Model file for the job. Use its own axes, mm. Face numbers are marked on the shaded views. A direction names the side the tool comes from. Round coordinates to 2 decimals unless told otherwise and drop trailing zeros. Loops run counter-clockwise (first coordinate to the right, second up) from the corner with the lowest first, then second, coordinate; pieces in that order, holes last. Notation, with made-up numbers: M 85,14.5 L 101,14.5 A17 cw 101,36.5 Z; hole C 78.5,47 d9. An arc over 180 degrees is marked long. Answer in a Markdown table with one row per item.
from build123d import *

# Parameters (mm, degrees)
MAIN_DEPTH                   = 24
SK_RECESS_R                  = 21
RECESS_DEPTH                 = 4
NUT_DEPTH                    = 83
SK_HOLE1_R                   = 2.5
HOLE1_DEPTH                  = 5
SK_HOLE_T_R                  = 4
HOLE_T_DEPTH                 = 17
SK_HOLE2_R                   = 4
HOLE2_DEPTH                  = 13
SK_HOLE3_R                   = 4
HOLE3_DEPTH                  = 16
SKETCH1_R                    = 3.3
THRUHOLES_DEPTH              = 113.841703284
SK_PRONG_GRV_W               = 8.5
SK_PRONG_GRV_H               = 119
PRONG_GRV_DEPTH              = 9
SK_HOLE4_R                   = 2.5
HOLE4_DEPTH                  = 5
GRV_REACH                    = 119.133
F_32_40SWITCHCHAMFER_SIZE    = 4.5
SKETCH5_W                    = 0.7
SKETCH5_H                    = 5
F_32_40SWITCHCUTDETAIL_DEPTH = 105.905910224
EXTRUDE1_START               = 5
SKETCH6_R                    = 2.5
EXTRUDE1_DEPTH               = 5
SKETCH9_R                    = 2.5
HOLE_5_DEPTH                 = 5


with BuildPart() as part:
    # sk-main → main (new, symmetric)
    with BuildSketch(Plane.XY):
        Polygon((0, -36), (83, -36), (83, 36), (0, 36), (0, 59.5), (-15, 59.5), (-15, -59.5), (0, -59.5), align=None)
    extrude(amount=MAIN_DEPTH, both=True)

    # sk-recess → recess (cut)
    with BuildSketch(Plane(origin=(83, 0, 0), x_dir=(0, 0, -1), z_dir=(1, 0, 0))):
        with Locations(Location((0, 0, 0), (0, 0, 90))):
            Circle(SK_RECESS_R)
    extrude(amount=-RECESS_DEPTH, mode=Mode.SUBTRACT)

    # sk-NUT → NUT (cut)
    with BuildSketch(Plane(origin=(83, 0, 0), x_dir=(0, 0, -1), z_dir=(1, 0, 0))):
        with BuildLine():
            Line((-21.622875656, 16.2), (-24, 16.2))
            Line((-24, 16.2), (-24, 13.2))
            Line((-24, 13.2), (-21.622875656, 13.2))
            ThreePointArc((-21.622875656, 13.2), (-18.3, 14.7), (-21.622875656, 16.2))
        make_face()
        with BuildLine():
            Line((-21.622875656, -13.2), (-24, -13.2))
            Line((-24, -13.2), (-24, -16.2))
            Line((-24, -16.2), (-21.622875656, -16.2))
            ThreePointArc((-21.622875656, -16.2), (-18.3, -14.7), (-21.622875656, -13.2))
        make_face()
        with BuildLine():
            Line((21.622875656, 13.2), (24, 13.2))
            Line((24, 13.2), (24, 16.2))
            Line((24, 16.2), (21.622875656, 16.2))
            ThreePointArc((21.622875656, 16.2), (18.3, 14.7), (21.622875656, 13.2))
        make_face()
        with BuildLine():
            Line((21.622875656, -13.2), (24, -13.2))
            Line((24, -13.2), (24, -16.2))
            Line((24, -16.2), (21.622875656, -16.2))
            ThreePointArc((21.622875656, -16.2), (18.3, -14.7), (21.622875656, -13.2))
        make_face()
    extrude(amount=-NUT_DEPTH, mode=Mode.SUBTRACT)

    # sk-hole1 → hole1 (cut)
    with BuildSketch(Plane(origin=(83, 0, 0), x_dir=(0, 0, -1), z_dir=(1, 0, 0))):
        with Locations(Location((-14, 29, 0), (0, 0, 90))):
            Circle(SK_HOLE1_R)
    extrude(amount=-HOLE1_DEPTH, mode=Mode.SUBTRACT)

    # sk-hole_t → hole_t (cut)
    with BuildSketch(Plane(origin=(83, 0, 0), x_dir=(0, 0, -1), z_dir=(1, 0, 0))):
        with Locations(Location((-16, -28, 0), (0, 0, 90))):
            Circle(SK_HOLE_T_R)
        with Locations(Location((16, 28, 0), (0, 0, 90))):
            Circle(SK_HOLE_T_R)
    extrude(amount=-HOLE_T_DEPTH, mode=Mode.SUBTRACT)

    # sk-hole2 → hole2 (cut)
    with BuildSketch(Plane(origin=(0, 36, 0), x_dir=(-1, 0, 0), z_dir=(0, 1, 0))):
        with Locations((-25, -16)):
            Circle(SK_HOLE2_R)
        with Locations((-25, 16)):
            Circle(SK_HOLE2_R)
    extrude(amount=-HOLE2_DEPTH, mode=Mode.SUBTRACT)

    # sk-hole3 → hole3 (cut)
    with BuildSketch(Plane(origin=(0, 0, -24), x_dir=(-1, 0, 0), z_dir=(0, 0, -1))):
        with Locations((-34, 28)):
            Circle(SK_HOLE3_R)
        with Locations((-34, -28)):
            Circle(SK_HOLE3_R)
    hole3 = extrude(amount=-HOLE3_DEPTH, mode=Mode.SUBTRACT)

    # Mirror1: hole3 across plane
    add(hole3.mirror(Plane.XY), mode=Mode.SUBTRACT)

    # Sketch1 → ThruHoles (cut, through all)
    with BuildSketch(Plane.XY.offset(24)):
        with Locations((34, 28)):
            Circle(SKETCH1_R)
        with Locations((34, -28)):
            Circle(SKETCH1_R)
    extrude(amount=-THRUHOLES_DEPTH, mode=Mode.SUBTRACT)

    # sk-prong_grv → prong_grv (cut, symmetric)
    with BuildSketch(Plane.XY):
        with Locations((-10.75, 0)):
            Rectangle(SK_PRONG_GRV_W, SK_PRONG_GRV_H)
    extrude(amount=PRONG_GRV_DEPTH, both=True, mode=Mode.SUBTRACT)

    # sk-hole4 → hole4 (cut)
    with BuildSketch(Plane.XZ.offset(36)):
        with Locations((45, 14)):
            Circle(SK_HOLE4_R)
        with Locations((71, -14)):
            Circle(SK_HOLE4_R)
    extrude(amount=-HOLE4_DEPTH, mode=Mode.SUBTRACT)

    # grv: up to this face of the body (flat: up to its plane)
    grv_end = Plane(part.part.faces().sort_by_distance((0, 47.75, 0))[0])
    # sk-grv → grv (cut, up to the picked face)
    with BuildSketch(Plane(origin=(83, 0, 0), x_dir=(0, 0, -1), z_dir=(1, 0, 0)), mode=Mode.PRIVATE) as grv_sk1:
        Polygon((-2.5, 36), (-2.5, 27.3), (-3.1, 27.020215405), (-3.1, 23), (3.1, 23), (3.1, 27.020215405), (2.5, 27.3), (2.5, 36), align=None)
    grv_tool1 = split(extrude(grv_sk1.sketch, amount=-GRV_REACH, mode=Mode.PRIVATE), bisect_by=grv_end, keep=Keep.BOTH, mode=Mode.PRIVATE)
    # sk-grv → grv (cut, up to the picked face)
    with BuildSketch(Plane(origin=(83, 0, 0), x_dir=(0, 0, -1), z_dir=(1, 0, 0)), mode=Mode.PRIVATE) as grv_sk2:
        Polygon((3.1, -23), (3.1, -27.020215405), (2.5, -27.3), (2.5, -36), (-2.5, -36), (-2.5, -27.3), (-3.1, -27.020215405), (-3.1, -23), align=None)
    grv_tool2 = split(extrude(grv_sk2.sketch, amount=-GRV_REACH, mode=Mode.PRIVATE), bisect_by=grv_end, keep=Keep.BOTH, mode=Mode.PRIVATE)
    add(grv_tool1.solids().sort_by(Axis((83, 29.184807, 0), (-1, 0, 0)))[0], mode=Mode.SUBTRACT)
    add(grv_tool2.solids().sort_by(Axis((83, -29.184807, 0), (-1, 0, 0)))[0], mode=Mode.SUBTRACT)

    # 32-40SwitchChamfer
    f_32_40switchchamfer_edges = [part.edges().sort_by_distance(p)[0] for p in [
        (41.5, 36, -2.5),
        (41.5, 36, 2.5),
        (41.5, -36, 2.5),
        (41.5, -36, -2.5),
    ]]
    chamfer(f_32_40switchchamfer_edges, length=F_32_40SWITCHCHAMFER_SIZE)

    # Sketch5 → 32-40SwitchCutDetail (cut, through all)
    with BuildSketch(Plane(origin=(0, 0, 0), x_dir=(0, 0, -1), z_dir=(1, 0, 0))):
        with Locations((-23.65, 14.7)):
            Rectangle(SKETCH5_W, SKETCH5_H)
        with Locations((23.65, 14.7)):
            Rectangle(SKETCH5_W, SKETCH5_H)
        with Locations((23.65, -14.7)):
            Rectangle(SKETCH5_W, SKETCH5_H)
        with Locations((-23.65, -14.7)):
            Rectangle(SKETCH5_W, SKETCH5_H)
    extrude(amount=F_32_40SWITCHCUTDETAIL_DEPTH, mode=Mode.SUBTRACT)

    # Sketch6 → Extrude1 (add)
    with BuildSketch(Plane.XZ.offset(31).offset(EXTRUDE1_START)):
        with Locations((71, -14)):
            Circle(SKETCH6_R)
    extrude(amount=-EXTRUDE1_DEPTH)

    # Sketch9 → Hole 5 (cut)
    with BuildSketch(Plane.XZ.offset(36)):
        with Locations((71, -14)):
            Circle(SKETCH9_R)
    extrude(amount=-HOLE_5_DEPTH, mode=Mode.SUBTRACT)


solid = part.part
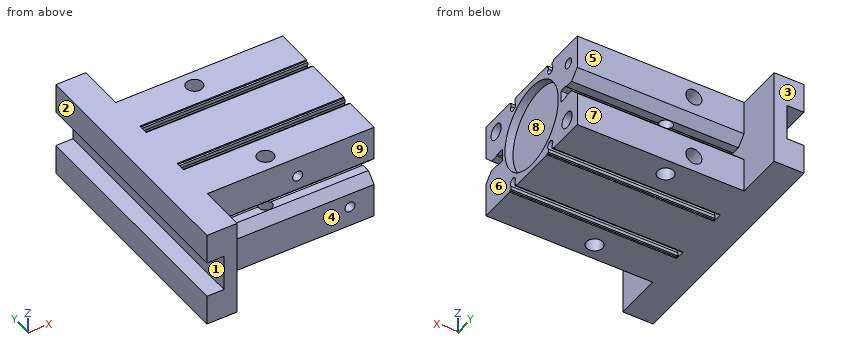
1. Saw through at A-A (z = 0). Write the cut outline in (x, y), and give its area (3 significant figures).
Verdict:
| item | result |
|---|---|
| outline | M -6.5,-59.5 L 0,-59.5 L 0,-23 L 83,-23 L 83,-21 L 79,-21 L 79,21 L 83,21 L 83,23 L 0,23 L 0,59.5 L -6.5,59.5 Z |
| area | 4,420 mm² |
2. Mould opens along Y. For the marked faces 6, 7, 8 and 9 say: +Y half, -Y half, draft (parallel to the pull), parting line (faces both ways), or undercut.
Verdict:
| item | result |
|---|---|
| face 6 | draft |
| face 7 | +Y half |
| face 8 | undercut |
| face 9 | -Y half |
3. Saw through at C-C (y = -50.5). Write the cut outline in (x, z), and give its area (3 significant figures).
Verdict:
| item | result |
|---|---|
| outline | M -15,-24 L 0,-24 L 0,24 L -15,24 L -15,9 L -6.5,9 L -6.5,-9 L -15,-9 Z |
| area | 567 mm² |
4. Saw through at B-B (x = 71). State how many separate pieces and enclosed holes the cut face has, and give its area (3 significant figures).
Verdict:
| item | result |
|---|---|
| separate pieces | 1 |
| enclosed holes | 2 |
| area | 3,070 mm² |
5. Tool access for the marked faces 1, 2, 3, 4 and 5: list every direction of +Z, -Z, +X, -X, +Y, -Y with a clear straight run to the whole face (end or side of a thin tool).
Verdict:
| item | result |
|---|---|
| face 1 | -X, +Y, -Y |
| face 2 | +Z, -Z, -X, +Y, -Y |
| face 3 | +Z, -Z, +X, -X, +Y |
| face 4 | +Z, -Z, +X, -Y |
| face 5 | +Z, -Z, +X, +Y |
6. Wall check: probe 1 along Z at (x, y) = (25, 30.5); probe 2 along Y at (x, z) = (34, -14.25); probe 3 along Z at (x, y) = (81.25, 0). Give the ranges that are in metal, low to high.
Verdict:
| item | result |
|---|---|
| probe 1 | z = -24 to -20, -12 to -2.5, 2.5 to 12, 20 to 24 |
| probe 2 | y = -36 to -32, -24 to 24, 32 to 36 |
| probe 3 | z = -24 to -21, 21 to 24 |
7. Pin check, flat tips, straight feed: pin 1 (1.5 mm diameter, centred on x = 1, z = 0.5, fed in from -Y); pin 2 (0.6 mm diameter, centred on x = 28.5, z = 23.5, fed in from -Y); pin 3 (2 mm diameter, centred on y = 44, z = -13.5, fed in from +X). Stop position of each tip, or through.
Verdict:
| item | result |
|---|---|
| pin 1 | stops at y = -23 |
| pin 2 | stops at y = -36 |
| pin 3 | stops at x = 0 |
